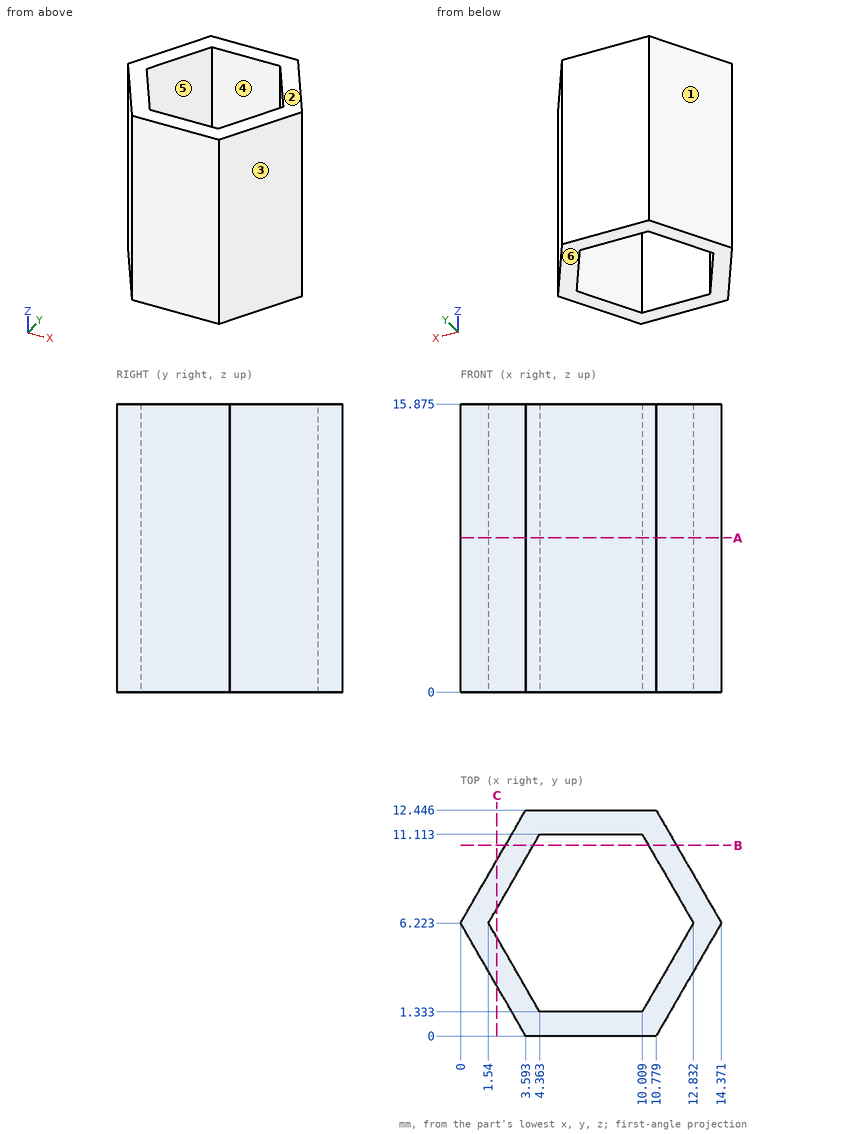
Geometry: see drawing. Coordinates: mm, zero at the bounding-box minimum. A direction names the side the tool comes from. Round coordinates to 2 decimals unless told otherwise and drop trailing zeros. Write each loop counter-clockwise with the first axis right and the second up, starting at its lowest first coordinate (ties: lowest second). Pieces come first, ordered by that corner, then holes.
Item 1: Mould query, pull axis X, two halves, no side actions, for the marked faces 1, 2, 3 and 4. Classes: +X half, -X half, draft (parallel to the pull), parting line (faces both ways), or undercut.
Item 2: Section query B-B (y = 10.5). Return loops of the section in (x, z) (1 decimal).
Item 3: Pin query (flat end, axial travel): P1, Ø6, axis at y = 6, z = 9.5, coming from the +X side. Return the tip coordinate at first contact, or that it passes through.
Item 4: Material intervals for L1, parallel to Y at x = 9.5, z = 12.75 (1 decimal); L2, parallel to X at y = 6.5, z = 6.25; L3, parallel to X at y = 5.25, z = 6.75, sorted ascending.
Item 5: Section query C-C (x = 2). Return loops of the section in (y, z) (1 decimal).
Item 6: Section query A-A (z = 8.5). Return loops of the section in (x, y) (1 decimal).
Item 7: Set-up query: the marked faces 5 and 6. Return all of +Z, -Z, +X, -X, +Y, -Y with unobstructed straight access to the full face (end or side cutting, diameter ignored); none if empty.
Completed:
1. face 1: -X half
1. face 2: draft
1. face 3: +X half
1. face 4: undercut
2. outline: (2.5, 0) - (4, 0) - (4, 15.9) - (2.5, 15.9) - close; (10.4, 0) - (11.9, 0) - (11.9, 15.9) - (10.4, 15.9) - close
3. P1: stops at x = 14.37
4. L1: y = 0 to 1.3, 11.1 to 12.4
4. L2: x = 0.16 to 1.7, 12.67 to 14.21
4. L3: x = 0.56 to 2.1, 12.27 to 13.81
5. outline: (2.8, 0) - (5.4, 0) - (5.4, 15.9) - (2.8, 15.9) - close; (7, 0) - (9.7, 0) - (9.7, 15.9) - (7, 15.9) - close
6. outline: (0, 6.2) - (3.6, 0) - (10.8, 0) - (14.4, 6.2) - (10.8, 12.4) - (3.6, 12.4) - close; hole (1.5, 6.2) - (4.4, 1.3) - (10, 1.3) - (12.8, 6.2) - (10, 11.1) - (4.4, 11.1) - close
7. face 5: +Z, -Z
7. face 6: -Z, +X, -X, +Y, -Y
